Read the model definition and answer for the solid it produces. Units are mm, in the model's axes. A direction names the side the tool comes from. Give positions to 0.01 mm unless a question says otherwise; leave off trailing zeros. Loops run counter-clockwise (first coordinate to the right, second up) from the corner with the lowest first, then second, coordinate; pieces in that order, holes last.
(1) Find section C-C, the plane y = 29. Write down the section's boundary in (x, z).
(2) Straight lines are drawn through the part: probe 1 along Z at (x, y) = (-60, 4.75); probe 2 along X at (y, z) = (58.5, -1); probe 3 along Z at (x, y) = (21.5, 36). For each, find the intervals that lie inside material, in ascending order.
(3) Find section B-B, the plane z = -14. Write down the section's boundary in (x, y).
(4) Find section D-D, the plane y = 16.5. Write down the section's boundary in (x, z), then the cut area to 3 significant figures.
(5) Determine the mould class of faces 5 (the face through (71.99, 6.08, 0.53)), 6 (the face through (1, 26, -30)), 7 (the face through (-6, 49, -1)) for opening direction X: pulls with the +X half, pulls with the -X half, needs draft (parallel to the pull), parting line crosses it, or undercut.
(6) Which of the six approach directions +Z, -Z, +X, -X, +Y, -Y give full straight-line access (tool end or side, diameter ignored) to faces 1 (the face through (-22.964, 27.725, -5.664)), 2 (the face through (0.794, 107.984, 9.46)), 3 (the face through (50, 12, 7)), 4 (the face through (17, 51, 18))?
(7) Find section A-A, the plane x = 0. Write down the section's boundary in (y, z), then the cut area to 3 significant figures.
(8) Each of these flat-tipped pins is pushed along its axis until it touches: P1, Ø1, axis at x = -31, z = -12, coming from the +Y side; P2, Ø8, axis at x = 54.5, z = 14, coming from the +Y side; P3, Ø2, axis at x = -1.5, z = 3.5, coming from the +Y side. Where does it stop, or does it pass through?
```python
from build123d import *

# Parameters (mm, degrees)
BOSS_EXTRUDE1_DEPTH = 30
FILLET1_R           = 30
FILLET2_R           = 30
SKETCH5_R           = 12
CUT_EXTRUDE1_DEPTH  = 98.857038582
FILLET3_RADIUS      = 30
FILLET3_LENGTH      = 12
SKETCH6_R           = 12
CUT_EXTRUDE2_DEPTH  = 98.857038582
SKETCH2_R           = 20
SKETCH2_R_2         = 12
BOSS_EXTRUDE2_DEPTH = 34
BOSS_EXTRUDE3_DEPTH = 12
BOSS_EXTRUDE4_DEPTH = 6


with BuildPart() as part:
    # Sketch1 → Boss-Extrude1 (new, symmetric)
    with BuildSketch(Plane.XY):
        with BuildLine():
            Line((-90, 0), (-24, 0))
            ThreePointArc((-24, 0), (0, 24), (24, 0))
            Line((24, 0), (90, 0))
            Line((90, 0), (90, 12))
            Line((90, 12), (33.941125497, 12))
            ThreePointArc((33.941125497, 12), (0, 36), (-33.941125497, 12))
            Line((-33.941125497, 12), (-90, 12))
            Line((-90, 12), (-90, 0))
        make_face()
    extrude(amount=BOSS_EXTRUDE1_DEPTH, both=True)

    # Fillet1
    fillet1_edges = [part.edges().sort_by_distance(p)[0] for p in [
        (90, 6, -30),
    ]]
    fillet(fillet1_edges, radius=FILLET1_R)

    # Fillet2
    fillet2_edges = [part.edges().sort_by_distance(p)[0] for p in [
        (90, 6, 30),
    ]]
    fillet(fillet2_edges, radius=FILLET2_R - 0.0001)  # a hair under: the kernel refuses the full size

    # Sketch5 → Cut-Extrude1 (cut, through all)
    with BuildSketch(Plane(origin=(0, 12, 0), x_dir=(1, 0, 0), z_dir=(0, 1, 0))):
        with Locations(Location((60, 0, 0), (0, 0, 180))):
            Circle(SKETCH5_R)
    extrude(amount=-CUT_EXTRUDE1_DEPTH, mode=Mode.SUBTRACT)

    # Fillet3: full round fillet: the end face becomes a half cylinder, R = half its width
    fillet3_face = Plane((-90, 6, 0), x_dir=(0, -1, 0), z_dir=(-1, 0, 0))  # on the end face: x along it, z out of the body
    fillet3_slab = fillet3_face.offset(-FILLET3_RADIUS / 2) * Box(FILLET3_LENGTH, 2 * FILLET3_RADIUS, FILLET3_RADIUS, mode=Mode.PRIVATE)  # the body's end, R deep
    fillet3_round = Plane((-60, 6, 0), x_dir=(-1, 0, 0), z_dir=(0, -1, 0)) * Cylinder(FILLET3_RADIUS, FILLET3_LENGTH, mode=Mode.PRIVATE)  # its axis R under the face
    add(fillet3_slab - fillet3_round, mode=Mode.SUBTRACT)

    # Sketch6 → Cut-Extrude2 (cut, through all)
    with BuildSketch(Plane(origin=(0, 12, 0), x_dir=(1, 0, 0), z_dir=(0, 1, 0))):
        with Locations(Location((-60, 0, 0), (0, 0, 180))):
            Circle(SKETCH6_R)
    extrude(amount=-CUT_EXTRUDE2_DEPTH, mode=Mode.SUBTRACT)



with BuildPart() as body_2:
    # Sketch2 → Boss-Extrude2 (new body)
    with BuildSketch(Plane.XY.offset(30)):
        with Locations((0, 88)):
            Circle(SKETCH2_R)
        with Locations((0, 88)):
            Circle(SKETCH2_R_2, mode=Mode.SUBTRACT)
    extrude(amount=-BOSS_EXTRUDE2_DEPTH)


with BuildPart() as part_1:
    add(part.part)

    add(body_2.part)  # Boss-Extrude3 merges body 2
    # Sketch3 → Boss-Extrude3 (add)
    with BuildSketch(Plane.XY.offset(30)):
        with BuildLine():
            Line((33.941125497, 12), (20, 88))
            ThreePointArc((20, 88), (0, 68), (-20, 88))
            Line((-20, 88), (-33.941125497, 12))
            ThreePointArc((-33.941125497, 12), (0, 36), (33.941125497, 12))
        make_face()
    extrude(amount=-BOSS_EXTRUDE3_DEPTH)

    # Sketch4 → Boss-Extrude4 (add, symmetric)
    with BuildSketch(Plane(origin=(0, 0, 0), x_dir=(0, 0, -1), z_dir=(1, 0, 0))):
        Polygon((-16.617348449, 30.307571786), (-22.191110534, 30.307571786), (-22.191110534, 71.304305049), (4, 71.304305049), (4, 68.110118748), (30, 36), (30, 30.307571786), align=None)
    extrude(amount=BOSS_EXTRUDE4_DEPTH, both=True)


solid = part_1.part
```
Entries:
1. outline: (-30.82, 18) - (-21.33, 18) - (-21.33, -30) - (21.33, -30) - (21.33, 18) - (30.82, 18) - (30.82, 30) - (-30.82, 30) - close
2. probe 1: z = -30 to -12, 12 to 30
2. probe 2: x = -6 to 6
2. probe 3: z = 18 to 30
3. outline: (-86.53, 0) - (-24, 0) arc R24 cw to (24, 0) - (86.53, 0) - (86.53, 12) - (33.94, 12) arc R36 ccw to (6, 35.5) - (6, 55.76) - (-6, 55.76) - (-6, 35.5) arc R36 ccw to (-33.94, 12) - (-86.53, 12) - close
4. outline: (-33.12, 18) - (-32, 18) - (-32, -30) - (-17.43, -30) - (-17.43, 30) - (-33.12, 30) - close; (17.43, -30) - (32, -30) - (32, 18) - (33.12, 18) - (33.12, 30) - (17.43, 30) - close
4. area: 1,770 mm2
5. face 5: undercut
5. face 6: needs draft
5. face 7: pulls with the -X half
6. face 1: -Z, -X
6. face 2: -Z
6. face 3: +Z, -Z, +X, +Y
6. face 4: -Z, +X
7. outline: (24, -30) - (36, -30) - (68.11, -4) - (76, -4) - (76, 30) - (24, 30) - close; (100, -4) - (108, -4) - (108, 30) - (100, 30) - close
7. area: 2,770 mm2
8. P1: stops at y = 19.12
8. P2: stops at y = 12
8. P3: stops at y = 107.99
